```python
from build123d import *

# Parameters (mm, degrees)
SKETCH1_R           = 15
BOSS_EXTRUDE1_DEPTH = 27
SKETCH2_R           = 19.07
BOSS_EXTRUDE2_DEPTH = 1.7
CUT_EXTRUDE1_DEPTH  = 40.382988713


with BuildPart() as part:
    # Sketch1 → Boss-Extrude1 (new body)
    with BuildSketch(Plane(origin=(0, 0, 0), x_dir=(1, 0, 0), z_dir=(0, 1, 0))):
        with Locations(Location((0, 0, 0), (0, 0, 270))):
            Circle(SKETCH1_R)
    extrude(amount=BOSS_EXTRUDE1_DEPTH)

    # Sketch2 → Boss-Extrude2 (add)
    with BuildSketch(Plane.XZ):
        with Locations(Location((0, 0, 0), (0, 0, 270))):
            Circle(SKETCH2_R)
    extrude(amount=BOSS_EXTRUDE2_DEPTH)

    # Sketch3 → Cut-Extrude1 (cut, through all)
    with BuildSketch(Plane.XZ.offset(1.7)):
        Polygon((-3.666174209, 6.35), (-7.332348419, 0), (-3.666174209, -6.35), (3.666174209, -6.35), (7.332348419, 0), (3.666174209, 6.35), align=None)
    extrude(amount=-CUT_EXTRUDE1_DEPTH, mode=Mode.SUBTRACT)


solid = part.part
```
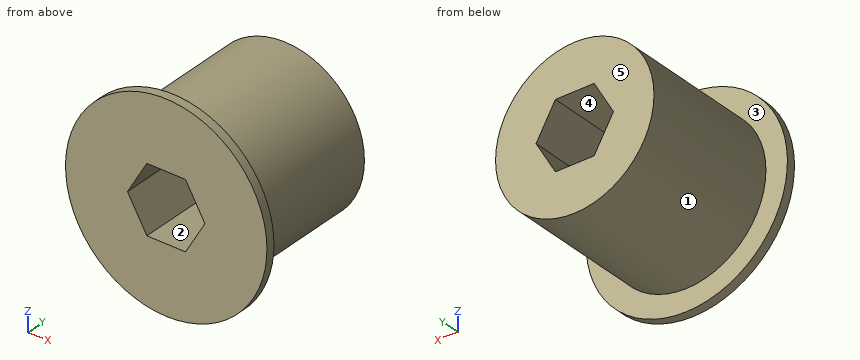
The model under review builds one solid part; all positions refer to its coordinate system, in mm. Face numbers are marked on the shaded views. A direction names the side the tool comes from. Coordinates: 2 decimals unless noted, no trailing zeros. Write each loop counter-clockwise with the first axis right and the second up, starting at its lowest first coordinate (ties: lowest second). Pieces come first, ordered by that corner, then holes. Notation, with made-up numbers: (-31.75, 13.5) -> (1.25, 13.5) arc R22 cw to (1.25, 48.5) -> close; hole circle Ø6 at (59.5, -38). An arc over 180 degrees is marked (long way). One line per item, written item: value. Start each with the question number.
Q1. Clearance check with flat-ended pins moving along their axes: P1, Ø1.5, axis at x = 12, y = 6.5, coming from the +Z side; P2, Ø10, axis at x = 12, y = 1.5, coming from the -Z side; P3, Ø4, axis at x = -3, y = 6.5, coming from the -Z side. State where each tip first meets the part, or that it passes through.
Q2. For the marked faces 4 and 5, list the 3-axis set-ups (+Z, -Z, +X, -X, +Y, -Y) from which the entire face can be reached by the end or side of a thin tool; tool diameter is ignored.
Q3. The part is to be moulded in two halves that separate along X. For the marked faces 1, 2 and 3, say which applies: +X half, -X half, draft (parallel to the pull), parting line (faces both ways), or undercut.
Q4. Add section B-B, the plane z = 1. Give the boundary of the cut face in (x, y) (3 decimals).
Q5. Add section C-C, the plane z = -13.5. Give the boundary of the cut face in (x, y).
Q6. Add section D-D, the plane x = 8. Give the boundary of the cut face in (y, z), then the cut area to 3 significant figures.
Q7. To check wall thickness, follow probe 1 along X at (y, z) = (4, -6); probe 2 along Z at (x, y) = (4.5, 13.75); probe 3 along X at (y, z) = (21.5, 4.5). State the ranges of each line that lie inside material, in increasing order.
Q8. Add section A-A, the plane x = 0. Give the boundary of the cut face in (y, z), then the cut area to 3 significant figures.
Response:
1. P1: z = 9.92
1. P2: z = -17.65
1. P3: z = -14.97
2. face 4: +Y, -Y
2. face 5: +Z, -Z, +X, -X, +Y
3. face 1: parting line
3. face 2: undercut
3. face 3: draft
4. outline: (-19.044, -1.7) -> (-6.755, -1.7) -> (-6.755, 27) -> (-14.967, 27) -> (-14.967, 0) -> (-19.044, 0) -> close; (6.755, -1.7) -> (19.044, -1.7) -> (19.044, 0) -> (14.967, 0) -> (14.967, 27) -> (6.755, 27) -> close
5. outline: (-13.47, -1.7) -> (13.47, -1.7) -> (13.47, 0) -> (6.54, 0) -> (6.54, 27) -> (-6.54, 27) -> (-6.54, 0) -> (-13.47, 0) -> close
6. outline: (-1.7, -17.31) -> (0, -17.31) -> (0, -12.69) -> (27, -12.69) -> (27, 12.69) -> (0, 12.69) -> (0, 17.31) -> (-1.7, 17.31) -> close
6. area: 744 mm²
7. probe 1: -13.75 to -3.87, 3.87 to 13.75
7. probe 2: -14.31 to -4.91, 4.91 to 14.31
7. probe 3: -14.31 to -4.73, 4.73 to 14.31
8. outline: (-1.7, -19.07) -> (0, -19.07) -> (0, -15) -> (27, -15) -> (27, -6.35) -> (-1.7, -6.35) -> close; (-1.7, 6.35) -> (27, 6.35) -> (27, 15) -> (0, 15) -> (0, 19.07) -> (-1.7, 19.07) -> close
8. area: 510 mm²
